Check sheet for the modelled part. Datum: model origin and axes. Units: mm. A direction names the side the tool comes from. Give positions to 0.01 mm unless a question says otherwise; leave off trailing zeros. Write each loop counter-clockwise with the first axis right and the second up, starting at its lowest first coordinate (ties: lowest second). Pieces come first, ordered by that corner, then holes. Notation, with made-up numbers: M 37,19.5 L 54,19.5 A24 ccw 54,57.5 Z; hole C -39,49 d6. An arc over 180 degrees is marked long. Write each question's results on one line, items separated by ' | '. Start each with the question number.
from build123d import *

# Parameters (mm, degrees)
F0_W     = 49.7362613678
F0_H     = 46.3653281331
F1_DEPTH = 2.54
F2_W     = 49.7362613678
F2_H     = 4.098245874
F3_DEPTH = 76.2
F4_W     = 3.7595648319
F4_H     = 23.1826640666
F4_H_2   = 23.9149127156
F5_DEPTH = 76.2


# Not quite as in the source:
# - the program builds the solid bodies; features that only make, move or delete a surface that nothing else refers to are left out


with BuildPart() as f1:
    # F0 (on Top) → F1 (new body)
    with BuildSketch(Plane.XY):
        with Locations((3.7595648319, -4.098245874)):
            Rectangle(F0_W, F0_H)
    extrude(amount=F1_DEPTH)

    # F2 (on face) → F3 (join)
    with BuildSketch(Plane.XY.offset(2.54)):
        with Locations((3.7595648319, -2.049122937)):
            Rectangle(F2_W, F2_H)
    extrude(amount=F3_DEPTH)

    # F4 (on face) → F5 (join)
    with BuildSketch(Plane.XY.offset(2.54)):
        with Locations((1.8797824159, -15.6895779073)):
            Rectangle(F4_W, F4_H)
        with Locations((1.8797824159, 7.8592104837)):
            Rectangle(F4_W, F4_H_2)
    extrude(amount=F5_DEPTH)


solid = f1.part
Q1. Section check A-A on y = 6. Record the boundary of the cut face in (x, z), plus the area to 3 significant figures.
Q2. Section check C-C on z = 28. Record the boundary of the cut face in (x, y).
Q3. Depth check by flat-ended pin: pin 1 Ø5 at (x, z) = (19.5, 62) entering from +Y; pin 2 Ø1.3 at (x, z) = (0, 1.5) entering from +Y; pin 3 Ø10 at (y, z) = (5.5, 15.5) entering from +X; pin 4 Ø12 at (y, z) = (-5.5, 62) entering from -X. Enter the tip coordinate at first touch or a pass-through.
Q4. Scan lines: L1, parallel to Y at x = -7, z = 70; L2, parallel to Z at x = 25.5, y = 0.5; L3, parallel to X at y = 5.5, z = 51. Record each from-to range of solid material in increasing order.
Q5. Tool access check on faces 1 (the face through (3.76, -16, 40)), 2 (the face through (28.628, -2, 28)), 3 (the face through (3.76, 10, 40)), 4 (the face through (0, -16, 40)), 5 (the face through (0, 10, 40)). Record the directions out of +Z, -Z, +X, -X, +Y, -Y that give a thin tool (end or side, any length) a straight path to the whole face; none if there is none.
Q6. Section check B-B on x = -13.5. Record the boundary of the cut face in (y, z), plus the area to 3 significant figures.
Check result:
1) outline: M -21.11,0 L 28.63,0 L 28.63,2.54 L 3.76,2.54 L 3.76,78.74 L 0,78.74 L 0,2.54 L -21.11,2.54 Z | area: 413 mm^2
2) outline: M -21.11,-4.1 L 0,-4.1 L 0,-27.28 L 3.76,-27.28 L 3.76,-4.1 L 28.63,-4.1 L 28.63,0 L 3.76,0 L 3.76,19.82 L 0,19.82 L 0,0 L -21.11,0 Z
3) pin 1: y = 0 | pin 2: y = 19.08 | pin 3: x = 3.76 | pin 4: x = -21.11
4) L1: -4.1 to 0 | L2: 0 to 2.54 | L3: 0 to 3.76
5) face 1: +Z, +X, -Y | face 2: +Z, -Z, +X, +Y, -Y | face 3: +Z, +X, +Y | face 4: +Z, -X, -Y | face 5: +Z, -X, +Y
6) outline: M -27.28,0 L 19.08,0 L 19.08,2.54 L 0,2.54 L 0,78.74 L -4.1,78.74 L -4.1,2.54 L -27.28,2.54 Z | area: 430 mm^2
